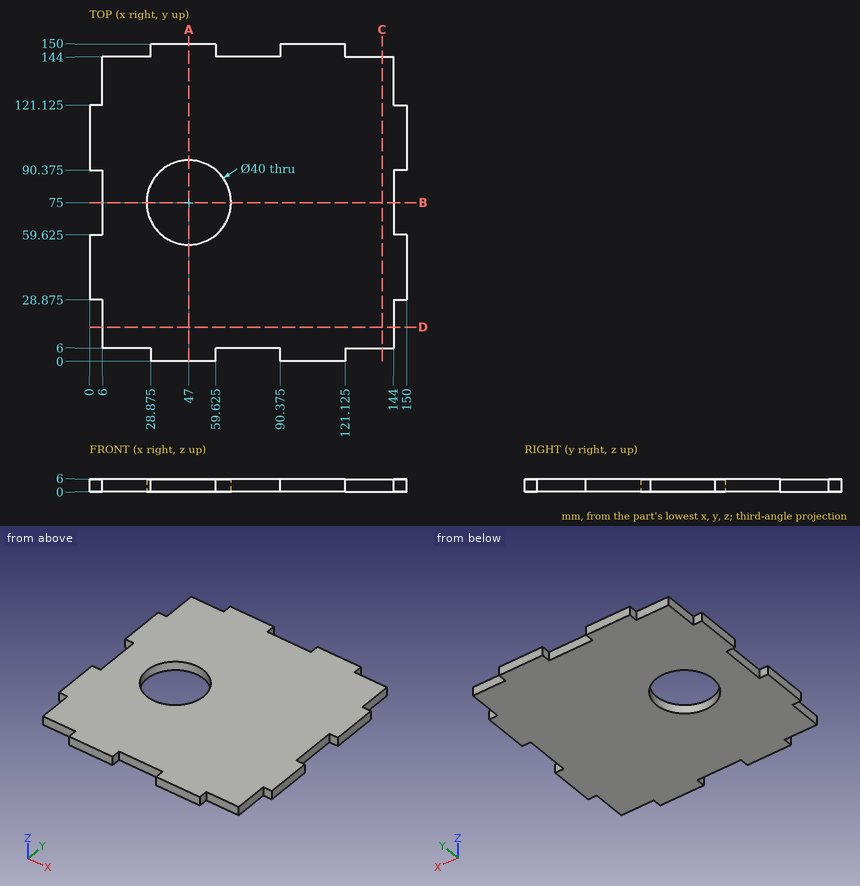
Input: dimensioned drawing with shaded views. Units: mm. Origin: part minimum x, y, z. Give positions to 0.01 mm unless a question says otherwise; leave off trailing zeros. Write each loop counter-clockwise with the first axis right and the second up, starting at its lowest first coordinate (ties: lowest second). Pieces come first, ordered by that corner, then holes. Notation, with made-up numbers: (10, -17) -> (22, -17) arc R17 ccw to (22, 11) -> close; hole circle Ø9 at (86.5, 79.25). An arc over 180 degrees is marked (long way). Answer as a JSON object with one key per item and string values.
1. Cut plane C-C on x = 138.5. Output: boundary loops of the cut face in (y, z).
Ans:
{"outline": "(6, 0) -> (144, 0) -> (144, 6) -> (6, 6) -> close"}
2. Contact query for flat-ended pins moving along their axis: pin 1 (3 mm diameter, centred on x = 4, z = 2, fed in from +Y) (3 decimals); pin 2 (1.8 mm diameter, centred on x = 13, z = 2.5, fed in from -Y); pin 3 (1.8 mm diameter, centred on y = 3, z = 4, fed in from -X) (3 decimals). Output: stop coordinate, or through.
Ans:
{"pin 1": "stops at y = 121.125", "pin 2": "stops at y = 6", "pin 3": "stops at x = 28.875"}
3. Cut plane B-B on y = 75. Output: boundary loops of the cut face in (x, z).
Ans:
{"outline": "(6, 0) -> (27, 0) -> (27, 6) -> (6, 6) -> close; (67, 0) -> (144, 0) -> (144, 6) -> (67, 6) -> close"}
4. Ray query, probe 1 along Y at (x, z) = (47, 1.6); probe 2 along Y at (x, z) = (77, 4.7); probe 3 along X at (y, z) = (82.5, 5.1). Return the intervals inside material, ascending. Write a range as from..to.
Ans:
{"probe 1": "y = 0..55, 95..150", "probe 2": "y = 6..144", "probe 3": "x = 6..28.46, 65.54..144"}
5. Cut plane A-A on x = 47. Output: boundary loops of the cut face in (y, z).
Ans:
{"outline": "(0, 0) -> (55, 0) -> (55, 6) -> (0, 6) -> close; (95, 0) -> (150, 0) -> (150, 6) -> (95, 6) -> close"}
